```python
from build123d import *

# Parameters (mm, degrees)
SKETCH1_R                = 16
SKETCH1_R_2              = 8
BOSS_EXTRUDE1_DEPTH      = 56
BOSS_EXTRUDE2_DEPTH      = 28
BOSS_EXTRUDE2_DEPTH_BACK = 28
SKETCH2_R                = 18
SKETCH2_R_2              = 8
SKETCH3_R                = 8
CUT_EXTRUDE1_DEPTH       = 73.221880507
SKETCH4_R                = 8
CUT_EXTRUDE2_DEPTH       = 87.994252854


with BuildPart() as part:
    # Sketch1 → Boss-Extrude1 (new body)
    with BuildSketch(Plane(origin=(0, 0, 0), x_dir=(1, 0, 0), z_dir=(0, 1, 0))):
        with Locations(Location((0, 0, 0), (0, 0, 270))):
            Circle(SKETCH1_R)
        with Locations(Location((0, 0, 0), (0, 0, 270))):
            Circle(SKETCH1_R_2, mode=Mode.SUBTRACT)
    extrude(amount=BOSS_EXTRUDE1_DEPTH)

    # Sketch2 → Boss-Extrude2 (add, two sides: drawn at the far end of the back side and taken through both)
    with BuildSketch(Plane.XY.offset(-BOSS_EXTRUDE2_DEPTH_BACK)):
        with Locations((18, 30.258098715)):
            Circle(SKETCH2_R)
        with Locations((18, 30.258098715)):
            Circle(SKETCH2_R_2, mode=Mode.SUBTRACT)
    extrude(amount=BOSS_EXTRUDE2_DEPTH + BOSS_EXTRUDE2_DEPTH_BACK)

    # Sketch3 → Cut-Extrude1 (cut, through all)
    with BuildSketch(Plane(origin=(0, 56, 0), x_dir=(1, 0, 0), z_dir=(0, 1, 0))):
        with Locations(Location((0, 0, 0), (0, 0, 270))):
            Circle(SKETCH3_R)
    extrude(amount=-CUT_EXTRUDE1_DEPTH, mode=Mode.SUBTRACT)

    # Sketch4 → Cut-Extrude2 (cut, through all)
    with BuildSketch(Plane.XY.offset(28)):
        with Locations((18, 30.258098715)):
            Circle(SKETCH4_R)
    extrude(amount=-CUT_EXTRUDE2_DEPTH, mode=Mode.SUBTRACT)


solid = part.part
```
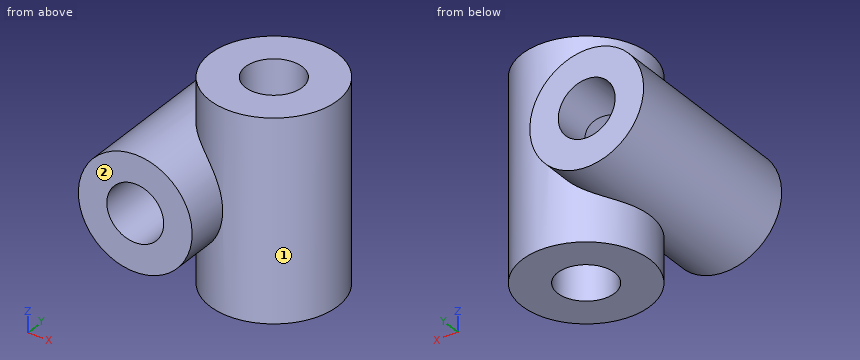
The listing builds one solid part. Answer for the finished solid, in the listing's coordinates (mm). Face numbers are marked on the shaded views. A direction names the side the tool comes from. Round coordinates to 2 decimals unless told otherwise and drop trailing zeros. Loops run counter-clockwise (first coordinate to the right, second up) from the corner with the lowest first, then second, coordinate; pieces in that order, holes last.
Q1. Section D-D, the plane z = 10 is taken. Determine the outline of the cut face in (x, y), then the cut area to 3 significant figures.
Q2. Find the intervals of material crossed by line 1 (Y direction, x = 18, z = 16.5); line 2 (Z direction, x = 0, y = 41); line 3 (X direction, y = 34, z = 0), in increasing order.
Q3. Section B-B, the plane z = 0 is taken. Determine the outline of the cut face in (x, y).
Q4. Given pin 1 Ø8 at (y, z) = (31, 6.5) entering from -X; pin 2 Ø6 at (x, z) = (3.5, 20) entering from -Y; pin 3 Ø12 at (x, z) = (9.5, 20.5) entering from -Y, each flat-ended and moving along its own axis, determine where each tip first touches the part or whether it passes through.
Q5. Section A-A, the plane x = 18 is taken. Determine the outline of the cut face in (y, z), then the cut area to 3 significant figures.
Q6. Which of the six approach directions +Z, -Z, +X, -X, +Y, -Y give full straight-line access (tool end or side, diameter ignored) to the marked faces 1 and 2?
Q7. Section C-C, the plane y = 14 is taken. Determine the outline of the cut face in (x, z), then the cut area to 3 significant figures.
Completed:
1. outline: (-12.49, 0) - (12.49, 0) - (12.49, 13.12) arc R18 ccw (long way) to (12.49, 47.39) - (12.49, 56) - (-12.49, 56) - close; hole circle Ø16 at (18, 30.26)
1. area: 1,900 mm2
2. line 1: y = 12.26 to 22.26, 38.26 to 48.26
2. line 2: z = -16 to -8, 8 to 16
2. line 3: x = -16 to -8, 8 to 10.93, 25.07 to 35.61
3. outline: (-16, 0) - (-8, 0) - (-8, 56) - (-16, 56) - close; (8, 0) - (16, 0) - (16, 12.37) arc R18 ccw (long way) to (16, 48.15) - (16, 56) - (8, 56) - close; hole circle Ø16 at (18, 30.26)
4. pin 1: stops at x = -15.8
4. pin 2: stops at y = 16.41
4. pin 3: stops at y = 12.43
5. outline: (12.26, -28) - (22.26, -28) - (22.26, 28) - (12.26, 28) - close; (38.26, -28) - (48.26, -28) - (48.26, 28) - (38.26, 28) - close
5. area: 1,120 mm2
6. face 1: none
6. face 2: +Z, -Z, +X, -X, -Y
7. outline: (10.28, -28) - (25.72, -28) - (25.72, 28) - (10.28, 28) - (10.28, 12.26) arc R16 ccw (long way) to (10.28, -12.26) - close; hole circle Ø16 at (0, 0)
7. area: 1,370 mm2
